Geometry check sheet. Reference: the model listing, model coordinates, mm. Coordinates: 2 decimals unless noted, no trailing zeros. Write each loop counter-clockwise with the first axis right and the second up, starting at its lowest first coordinate (ties: lowest second). Pieces come first, ordered by that corner, then holes. Notation, with made-up numbers: (48.5, 67.5) -> (90.5, 67.5) arc R18 cw to (90.5, 81.5) -> close; hole circle Ø2 at (-4, 17). An arc over 180 degrees is marked (long way). One line per question, with ' | ' between items.
from build123d import *

# Parameters (mm, degrees)
SKETCH3_R               = 3.175
BOSS_EXTRUDE1_DEPTH     = 304.8
CHAMFER1_SIZE           = 0.635
CUT_EXTRUDE1_START      = -92.927050112
SKETCH4_R               = 3.175
CUT_EXTRUDE1_DEPTH      = 517.672949888
SKETCH5_R               = 0.5953125
CUT_EXTRUDE2_DEPTH      = 4.175
CUT_EXTRUDE2_DEPTH_BACK = 4.175


with BuildPart() as part:
    # Sketch3 → Boss-Extrude1 (new body, symmetric)
    with BuildSketch(Plane.XY):
        Circle(SKETCH3_R)
    extrude(amount=BOSS_EXTRUDE1_DEPTH, both=True)

    # Chamfer1
    chamfer1_edges = [part.edges().sort_by_distance(p)[0] for p in [
        (-3.175, 0, -304.8),
        (-3.175, 0, 304.8),
    ]]
    chamfer(chamfer1_edges, length=CHAMFER1_SIZE)

    # Sketch4 → Cut-Extrude1 (cut, through all)
    with BuildSketch(Plane.XY.offset(304.8).offset(CUT_EXTRUDE1_START)):
        Circle(SKETCH4_R)
    extrude(amount=-CUT_EXTRUDE1_DEPTH, mode=Mode.SUBTRACT)

    # Sketch5 → Cut-Extrude2 (cut, two sides)
    with BuildSketch(Plane(origin=(0, 0, 0), x_dir=(1, 0, 0), z_dir=(0, 1, 0))) as cut_extrude2_sk:
        with Locations((0, -213.460449888)):
            Circle(SKETCH5_R)
        with Locations((0, -303.2125)):
            Circle(SKETCH5_R)
    extrude(amount=CUT_EXTRUDE2_DEPTH, mode=Mode.SUBTRACT)
    extrude(cut_extrude2_sk.sketch, amount=-CUT_EXTRUDE2_DEPTH_BACK, mode=Mode.SUBTRACT)


solid = part.part
1. Go/stop test with a flat-tipped pin: P1, Ø1, axis at x = 0, z = 303.21, coming from the -Y side. Record where the tip stops, or that it passes through.
Worked answers:
P1: through
2. Cross-section at A-A on z = 254. Record the boundary of the cut face in (x, y) (3 decimals), and give its area (3 significant figures).
Worked answers:
outline: circle Ø6.35 at (0, 0) | area: 31.7 mm²
3. Material ranges on line 1 (Z direction, x = 0, y = 0.9); line 2 (Z direction, x = 0.5, y = 2.75); line 3 (X direction, y = 0.25, z = 237), recorded low to high. Write a range as from..to.
Worked answers:
line 1: 211.87..212.87, 214.06..302.62, 303.81..304.8 | line 2: 211.87..213.14, 213.78..302.89, 303.54..304.54 | line 3: -3.17..3.17
